Geometry: final body of the model. Coordinates: model frame, mm. Face numbers are marked on the shaded views. A direction names the side the tool comes from. Coordinates: 2 decimals unless noted, no trailing zeros. Write each loop counter-clockwise with the first axis right and the second up, starting at its lowest first coordinate (ties: lowest second). Pieces come first, ordered by that corner, then holes.
from build123d import *

# Parameters (mm, degrees)
SKETCH_1_W          = 35
SKETCH_1_H          = 180
EXTRUDE_1_DEPTH     = 10
SKETCH_2_W          = 22
SKETCH_2_H          = 39
CUT_EXTRUDE_1_DEPTH = 39
FILLET_1_R          = 4
SKETCH_3_R          = 1.65
CUT_EXTRUDE_2_DEPTH = 15
SKETCH_5_R          = 1.65
CUT_EXTRUDE_3_DEPTH = 15
SKETCH_6_R          = 1.139472941
SKETCH_6_R_2        = 1.207913295
CUT_EXTRUDE_4_DEPTH = 12
SKETCH_7_R          = 1.65
CUT_EXTRUDE_5_DEPTH = 12


with BuildPart() as part:
    # Эскиз1 → Бобышка-Вытянуть1 (new body)
    with BuildSketch(Plane.XY):
        with Locations((-10.704653715, -21.244958968)):
            Rectangle(SKETCH_1_W, SKETCH_1_H)
    extrude(amount=EXTRUDE_1_DEPTH)

    # Эскиз2 → Вырез-Вытянуть1 (cut)
    with BuildSketch(Plane(origin=(0, 0, 0), x_dir=(-1, 0, 0), z_dir=(0, 0, -1))):
        with Locations((4.204653715, 19.255041032)):
            Rectangle(SKETCH_2_W, SKETCH_2_H)
    extrude(amount=-CUT_EXTRUDE_1_DEPTH, mode=Mode.SUBTRACT)

    # Скругление1
    fillet_1_edges = [part.edges().sort_by_distance(p)[0] for p in [
        (-15.204653715, 38.755041032, 5),
        (-15.204653715, -0.244958968, 5),
    ]]
    fillet(fillet_1_edges, radius=FILLET_1_R)

    # Эскиз3 → Вырез-Вытянуть2 (cut)
    with BuildSketch(Plane.ZY.offset(28.204653715)):
        with Locations(Location((5, 38.651818595, 0), (0, 0, 270))):
            Circle(SKETCH_3_R)
        with Locations(Location((5, -21.348181405, 0), (0, 0, 270))):
            Circle(SKETCH_3_R)
        with Locations(Location((5, -81.348181405, 0), (0, 0, 270))):
            Circle(SKETCH_3_R)
    extrude(amount=-CUT_EXTRUDE_2_DEPTH, mode=Mode.SUBTRACT)

    # Эскиз5 → Вырез-Вытянуть3 (cut)
    with BuildSketch(Plane(origin=(6.795346285, 0, 0), x_dir=(0, 0, -1), z_dir=(1, 0, 0))):
        with Locations(Location((-5, 53.755041032, 0), (0, 0, 90))):
            Circle(SKETCH_5_R)
        with Locations(Location((-5, -26.244958968, 0), (0, 0, 90))):
            Circle(SKETCH_5_R)
        with Locations(Location((-5, -96.244958968, 0), (0, 0, 90))):
            Circle(SKETCH_5_R)
    extrude(amount=-CUT_EXTRUDE_3_DEPTH, mode=Mode.SUBTRACT)

    # Эскиз6 → Вырез-Вытянуть4 (cut)
    with BuildSketch(Plane.XZ.offset(111.244958968)):
        with Locations(Location((-22.204653715, 5, 0), (0, 0, 270))):
            Circle(SKETCH_6_R)
        with Locations(Location((-3.204653715, 5, 0), (0, 0, 270))):
            Circle(SKETCH_6_R_2)
    extrude(amount=-CUT_EXTRUDE_4_DEPTH, mode=Mode.SUBTRACT)

    # Эскиз7 → Вырез-Вытянуть5 (cut)
    with BuildSketch(Plane(origin=(0, 68.755041032, 0), x_dir=(1, 0, 0), z_dir=(0, 1, 0))):
        with Locations(Location((-21.204653715, -5, 0), (0, 0, 270))):
            Circle(SKETCH_7_R)
    extrude(amount=-CUT_EXTRUDE_5_DEPTH, mode=Mode.SUBTRACT)


solid = part.part
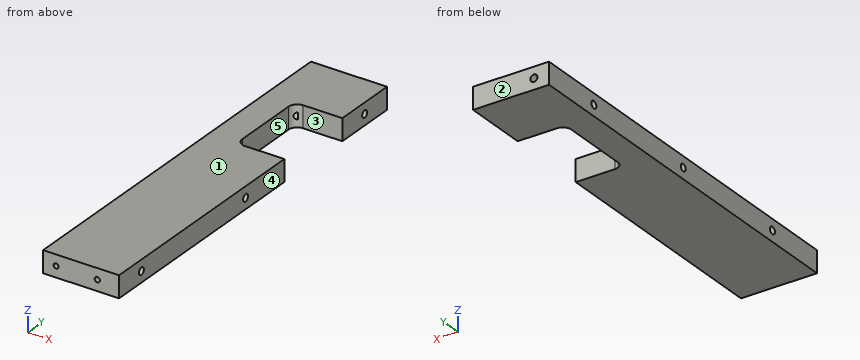
Item 1: Pin query (flat end, axial travel): pin 1 (3 mm diameter, centred on y = -81.35, z = 5, fed in from -X); pin 2 (0.7 mm diameter, centred on x = -3, z = 5, fed in from -Y); pin 3 (12 mm diameter, centred on x = -3.5, y = 19.5, fed in from -Z); pin 4 (1 mm diameter, centred on y = -27, z = 4.5, fed in from +X). Return the tip coordinate at first contact, or that it passes through.
Derived:
pin 1: stops at x = -13.2
pin 2: stops at y = -99.24
pin 3: passes through
pin 4: stops at x = -8.2
Item 2: Material intervals for probe 1 along X at (y, z) = (-107, 5); probe 2 along Y at (x, z) = (-5, 3); probe 3 along Y at (x, z) = (4, 4), sorted ascending.
Derived:
probe 1: x = -28.2 to -23.34, -21.07 to -4.41, -2 to 6.8
probe 2: y = -111.24 to -0.24, 38.76 to 68.76
probe 3: y = -111.24 to -97.56, -94.93 to -27.56, -24.93 to -0.24, 38.76 to 52.44, 55.07 to 68.76
Item 3: Set-up query: the marked faces 4 and 5. Return all of +Z, -Z, +X, -X, +Y, -Y with unobstructed straight access to the full face (end or side cutting, diameter ignored); none if empty.
Derived:
face 4: +Z, -Z, +X, +Y, -Y
face 5: +Z, -Z, +X
Item 4: Pull-direction query (Y, two-part tool) for the marked faces 1, 2 and 3; classes: released by +Y, released by -Y, zero draft, split by the parting line, or undercut.
Derived:
face 1: zero draft
face 2: released by +Y
face 3: undercut
Item 5: Section A-A, the plane x = 2. Output: boundary loops of the cut face in (y, z), plus the area to 3 significant figures.
Derived:
outline: (-111.24, 0) - (-0.24, 0) - (-0.24, 10) - (-111.24, 10) - close; (38.76, 0) - (68.76, 0) - (68.76, 10) - (38.76, 10) - close; hole circle Ø3.3 at (-96.24, 5); hole circle Ø3.3 at (-26.24, 5); hole circle Ø3.3 at (53.76, 5)
area: 1,380 mm2
